from build123d import *

# Parameters (mm, degrees)
EXTRUSION1_DEPTH        = 38
ESQUISSE2_R             = 2.8
ENL_V_MAT_EXTRU_1_DEPTH = 39
CONG_1_R                = 0.5
CONG_2_R                = 1


with BuildPart() as part:
    # Esquisse1 → Extrusion1 (new body)
    with BuildSketch(Plane.XY):
        Polygon((-2.8, 11), (-2.8, 9.3), (-8.097918472, 9.3), (-3.297918472, 4.5), (3.297918472, 4.5), (8.097918472, 9.3), (2.8, 9.3), (2.8, 11), (11, 11), (11, 2.8), (9.3, 2.8), (9.3, 8.097918472), (4.5, 3.297918472), (4.5, -3.297918472), (9.3, -8.097918472), (9.3, -2.8), (11, -2.8), (11, -11), (2.8, -11), (2.8, -9.3), (8.097918472, -9.3), (3.297918472, -4.5), (-3.297918472, -4.5), (-8.097918472, -9.3), (-2.8, -9.3), (-2.8, -11), (-11, -11), (-11, -2.8), (-9.3, -2.8), (-9.3, -8.097918472), (-4.5, -3.297918472), (-4.5, 3.297918472), (-9.3, 8.097918472), (-9.3, 2.8), (-11, 2.8), (-11, 11), align=None)
    extrude(amount=EXTRUSION1_DEPTH)

    # Esquisse2 → Enlèv. mat.-Extru.1 (cut, through all)
    with BuildSketch(Plane(origin=(0, 0, 0), x_dir=(-1, 0, 0), z_dir=(0, 0, -1))):
        Circle(ESQUISSE2_R)
    extrude(amount=-ENL_V_MAT_EXTRU_1_DEPTH, mode=Mode.SUBTRACT)

    # Congé1
    cong_1_edges = [part.edges().sort_by_distance(p)[0] for p in [
        (-11, 11, 19),
        (11, 11, 19),
        (11, -11, 19),
        (-11, -11, 19),
    ]]
    fillet(cong_1_edges, radius=CONG_1_R)

    # Congé2
    cong_2_edges = [part.edges().sort_by_distance(p)[0] for p in [
        (-4.5, -3.297918472, 19),
        (-4.5, 3.297918472, 19),
        (-3.297918472, 4.5, 19),
        (3.297918472, 4.5, 19),
        (4.5, 3.297918472, 19),
        (4.5, -3.297918472, 19),
        (3.297918472, -4.5, 19),
        (-3.297918472, -4.5, 19),
    ]]
    fillet(cong_2_edges, radius=CONG_2_R)


solid = part.part
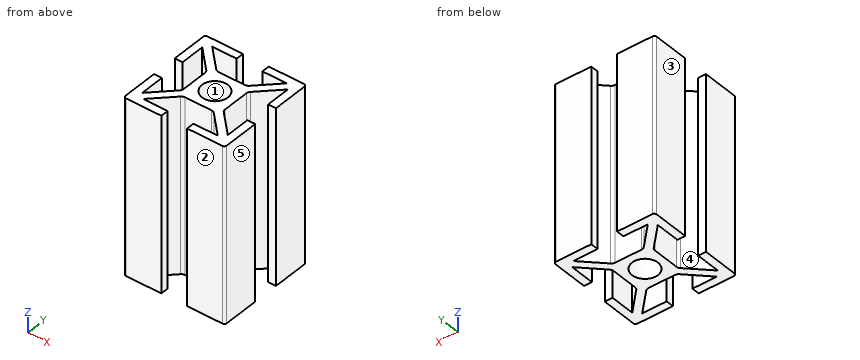
Build history of the part. All positions in model axes, mm. Face numbers are marked on the shaded views. A direction names the side the tool comes from. Round coordinates to 2 decimals unless told otherwise and drop trailing zeros. Loops run counter-clockwise (first coordinate to the right, second up) from the corner with the lowest first, then second, coordinate; pieces in that order, holes last. Notation, with made-up numbers: (43.5, -13) -> (97.5, -13) arc R18 ccw to (97.5, 8) -> close; hole circle Ø11 at (-36, -29.75). An arc over 180 degrees is marked (long way). One line per item, written item: value. Start each with the question number.
Q1. Drop a flat-ended pin along its axis: pin 1 Ø3 at (x, z) = (-0.5, 11) entering from +Y. Give the stop position or say it passes through.
Q2. 3-axis set-ups, long thin cutter, end or side, ignore diameter. For the marked faces 4 and 5: which of +Z, -Z, +X, -X, +Y, -Y reach the whole face in a straight line?
Q3. Probe line 1 along Y through (x, z) = (0, 16.5); line 2 along X through (y, z) = (4.75, 14.5); line 3 along X through (y, z) = (3.25, 6). List the from-to ranges inside material, lowest first.
Q4. Cut at A-A on y = 0. List the corners of the cut face in (x, z).
Q5. Cut at C-C on x = 6.5. List the corners of the cut face in (y, z), plus the area to 3 significant figures.
Q6. Two-plate mould, pull along X, no slides. Class the marked faces 1, 2 and 3: released by +X, released by -X, zero draft, split by the parting line, or undercut.
Computed:
1. pin 1: y = 4.5
2. face 4: +Z, -Z
2. face 5: +Z, -Z, +X, +Y, -Y
3. line 1: -4.5 to -2.8, 2.8 to 4.5
3. line 2: -11 to -9.3, -5.95 to -3.55, 3.55 to 5.95, 9.3 to 11
3. line 3: -11 to -9.3, -4.57 to 4.57, 9.3 to 11
4. outline: (-4.5, 0) -> (-2.8, 0) -> (-2.8, 38) -> (-4.5, 38) -> close; (2.8, 0) -> (4.5, 0) -> (4.5, 38) -> (2.8, 38) -> close
5. outline: (-11, 0) -> (-9.3, 0) -> (-9.3, 38) -> (-11, 38) -> close; (-7.7, 0) -> (-5.3, 0) -> (-5.3, 38) -> (-7.7, 38) -> close; (5.3, 0) -> (7.7, 0) -> (7.7, 38) -> (5.3, 38) -> close; (9.3, 0) -> (11, 0) -> (11, 38) -> (9.3, 38) -> close
5. area: 312 mm²
6. face 1: undercut
6. face 2: zero draft
6. face 3: released by -X
